The listing builds one solid part. Answer for the finished solid, in the listing's coordinates (mm). A direction names the side the tool comes from. Give positions to 0.01 mm unless a question says otherwise; leave off trailing zeros. Write each loop counter-clockwise with the first axis right and the second up, starting at its lowest first coordinate (ties: lowest second). Pieces come first, ordered by that corner, then holes. Notation, with made-up numbers: (38.5, 15.5) -> (46.5, 15.5) arc R20 cw to (46.5, 20.5) -> close; hole circle Ø3 at (-35, 22). An arc over 180 degrees is marked (long way). Put each result on its own line as item: value. Start each with the question number.
1) A flat-ended cylindrical pin translates along its axis: pin 1 Ø2 at (x, z) = (214.5, 167.5) entering from -Y. Find the tip coordinate at first contact, or state that the pin passes through.
2) A cutting plane is placed at B-B (x = 125). Write down the section's boundary in (y, z).
3) A cutting plane is placed at D-D (y = 10). Write down the section's boundary in (x, z), then the cut area to 3 significant figures.
4) For a pull along X with two mould halves and no side action, classify faces 1 (the flat face through (25, -74, 123)), 2 (the flat face through (127, 15, 250)), 3 (the flat face through (250, -51, 123)), 4 (the flat face through (0, -51, 127)) as released by +X, released by -X, zero draft, split by the parting line, or undercut.
5) Find the intervals of material crossed by line 1 along Z through (x, y) = (125, 19); line 2 along X through (y, z) = (-92, 15.5); line 3 along Y through (x, z) = (93.5, 69.5), in increasing order. Write a range as from..to.
6) For faces 5 (the cylindrical face through (106.574, 24.65, 141.896)), 6 (the flat face through (225, -74, 127)), determine the directions among +Z, -Z, +X, -X, +Y, -Y from which every point of the face is accessible in a straight line to the end or side of a thin tool.
7) A cutting plane is placed at C-C (y = -12). Write down the section's boundary in (x, z), then the cut area to 3 significant figures.
8) A cutting plane is placed at A-A (z = 125). Write down the section's boundary in (x, y), then the cut area to 3 significant figures.
Autodesk Fusion 360 part; units mm, degrees
sketch "Sketch1" plane through (0, 0, 0) normal (0, 1, 0) x (1, 0, 0)
  line L0 (0, 0) -> (100, 0)
  line L1 (100, 0) -> (100, -100)
  line L2 (100, -100) -> (0, -100)
  line L3 (0, -100) -> (0, 0)
  dimension "d1" = 100
  dimension "d2" = 100
extrude "Extrude1" add sketch "Sketch1" along normal blind 20
sketch "Sketch2" plane through (0, 0, 0) normal (0, -1, 0) x (1, 0, 0)
  line L0 (100, 100) -> (0, 100)
  line L1 (0, 100) -> (0, 0)
  line L2 (0, 0) -> (100, 0)
  line L3 (100, 0) -> (100, 100)
  line L4 (10, 100) -> (90, 100)
  line L5 (90, 100) -> (90, 0)
  line L6 (90, 0) -> (10, 0)
  line L7 (10, 0) -> (10, 100)
  dimension "d5" = 10
  dimension "d6" = 80
extrude "Extrude2" add sketch "Sketch2" along normal blind 60 contours L0 L2 L3 L5 | L0 L1 L2 L7
sketch "Sketch3" plane through (0, 0, 0) normal (0, -1, 0) x (1, 0, 0)
  line L0 (10, 100) -> (10, 0)
  line L1 (10, 0) -> (90, 0)
  line L2 (90, 0) -> (90, 100)
  line L3 (90, 100) -> (10, 100)
  circle A0 centre (50, 50) radius 10
  dimension "d9" = 20
extrude "Extrude3" cut sketch "Sketch3" against normal blind 20 contours A0
scale "Scale1" factor 2.5 about (0, 0, 0) bodies 1
Reply:
1. pin 1: stops at y = 0
2. outline: (0, 0) -> (50, 0) -> (50, 100) -> (0, 100) -> close; (0, 150) -> (50, 150) -> (50, 250) -> (0, 250) -> close
3. outline: (0, 0) -> (250, 0) -> (250, 250) -> (0, 250) -> close; hole circle Ø50 at (125, 125)
3. area: 60,500 mm2
4. face 1: undercut
4. face 2: zero draft
4. face 3: released by +X
4. face 4: released by -X
5. line 1: z = 0..100, 150..250
5. line 2: x = 0..25, 225..250
5. line 3: y = 0..50
6. face 5: +Y, -Y
6. face 6: +Z, -Z, -Y
7. outline: (0, 0) -> (25, 0) -> (25, 250) -> (0, 250) -> close; (225, 0) -> (250, 0) -> (250, 250) -> (225, 250) -> close
7. area: 12,500 mm2
8. outline: (0, -150) -> (25, -150) -> (25, 0) -> (100, 0) -> (100, 50) -> (0, 50) -> close; (150, 0) -> (225, 0) -> (225, -150) -> (250, -150) -> (250, 50) -> (150, 50) -> close
8. area: 17,500 mm2
